Answer from the drawing. Dimensions are ordinates in mm from the lowest x, y and z of the part. A direction names the side the tool comes from. Coordinates: 2 decimals unless noted, no trailing zeros. Order: outer loops, then holes, each group sorted by start corner. A loop starts at its lowest first (then second) coordinate and runs counter-clockwise, first axis right, second up. Notation, with made-up numbers: M 47.25,22 L 69.25,22 A25 ccw 69.25,56 Z; hole C 81.5,-8.75 d7. An arc over 180 degrees is marked long. Write each question's results on one line, items separated by ' | '.
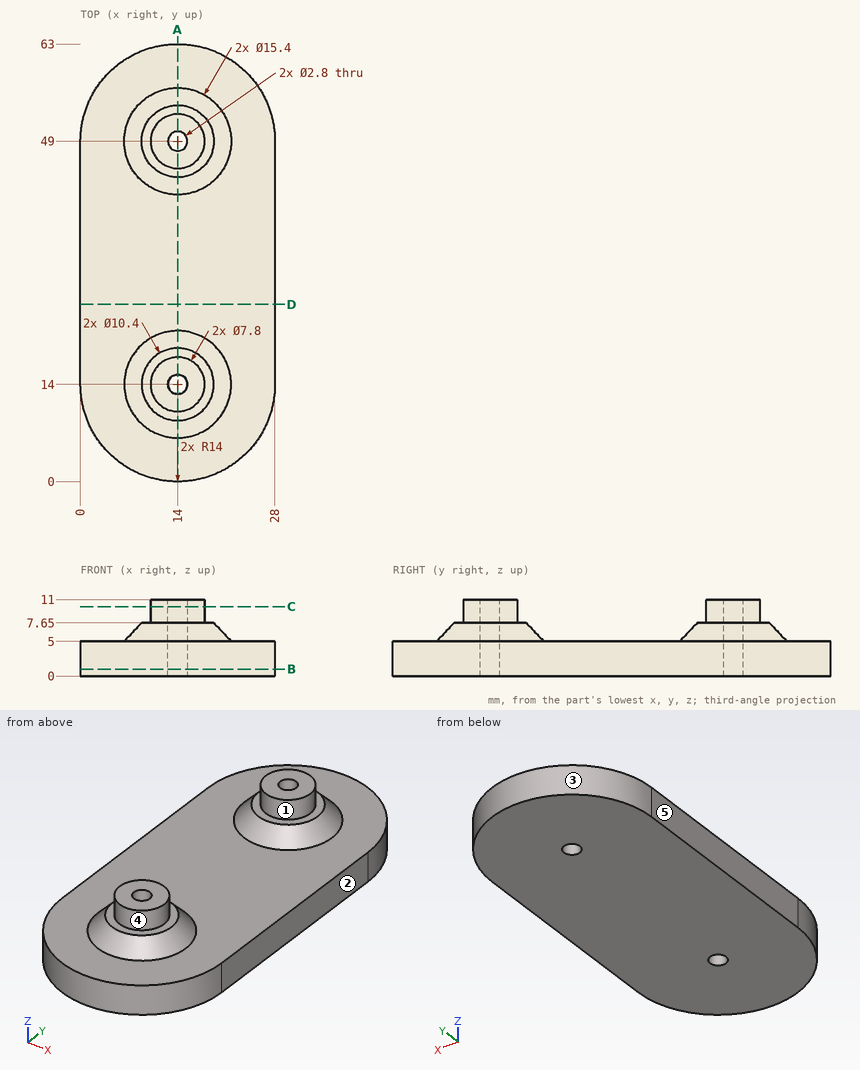
(1) The part is cut by section A-A, the plane x = 14. Write down the section's boundary in (y, z).
Conclusion:
outline: M 0,0 L 12.6,0 L 12.6,11 L 10.1,11 L 10.1,7.65 L 8.8,7.65 L 6.3,5 L 0,5 Z; M 15.4,0 L 47.6,0 L 47.6,11 L 45.1,11 L 45.1,7.65 L 43.8,7.65 L 41.3,5 L 21.7,5 L 19.2,7.65 L 17.9,7.65 L 17.9,11 L 15.4,11 Z; M 50.4,0 L 63,0 L 63,5 L 56.7,5 L 54.2,7.65 L 52.9,7.65 L 52.9,11 L 50.4,11 Z
(2) The part is cut by section B-B, the plane z = 1. Write down the section's boundary in (x, y), then the cut area to 3 significant figures.
Conclusion:
outline: M 0,14 A14 ccw 28,14 L 28,49 A14 ccw 0,49 Z; hole C 14,14 d2.8; hole C 14,49 d2.8 | area: 1,580 mm²
(3) The part is cut by section D-D, the plane y = 25.5. Write down the section's boundary in (x, z).
Conclusion:
outline: M 0,0 L 28,0 L 28,5 L 0,5 Z
(4) The part is cut by section C-C, the plane z = 10. Write down the section's boundary in (x, y), then the cut area to 3 significant figures.
Conclusion:
outline: C 14,14 d7.8; C 14,49 d7.8; hole C 14,14 d2.8; hole C 14,49 d2.8 | area: 83.3 mm²
(5) For the marked faces 4 and 5, determine the directions among +Z, -Z, +X, -X, +Y, -Y from which every point of the face is accessible in a straight line to the end or side of a thin tool.
Conclusion:
face 4: +Z | face 5: +Z, -Z, -X, +Y, -Y
(6) Given pin 1 (8.5 mm diameter, centred on x = 15, y = 28.5, fed in from +Z); pin 2 (4 mm diameter, centred on x = 15.5, z = 8, fed in from -Y), each flat-ended and moving along its own axis, determine where each tip first touches the part or whether it passes through.
Conclusion:
pin 1: z = 5 | pin 2: y = 7.37
(7) Straight lines are drawn through the part: line 1 (Y direction, x = 14, z = 3.25); line 2 (Y direction, x = 14.75, z = 6.75); line 3 (X direction, y = 14, z = 3.75). For each, find the intervals that lie inside material, in ascending order.
Conclusion:
line 1: 0 to 12.6, 15.4 to 47.6, 50.4 to 63 | line 2: 8 to 12.82, 15.18 to 20, 43 to 47.82, 50.18 to 55 | line 3: 0 to 12.6, 15.4 to 28
(8) The mould has two halves that part along Y. Classify the marked faces 1, 2 and 3: pulls with the +Y half, pulls with the -Y half, needs draft (parallel to the pull), parting line crosses it, or undercut.
Conclusion:
face 1: undercut | face 2: needs draft | face 3: pulls with the +Y half
